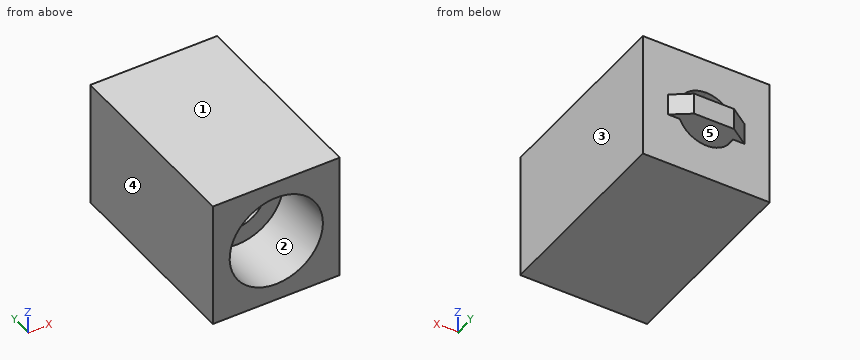
```python
from build123d import *

# Parameters (mm, degrees)
SKETCH1_R           = 12.7
BOSS_EXTRUDE1_DEPTH = 38.1
SKETCH2_R           = 5.715
CUT_EXTRUDE1_DEPTH  = 43.121134838
SKETCH3_R           = 9.3345
CUT_EXTRUDE2_DEPTH  = 12.7
SKETCH4_R           = 12.7
SKETCH4_R_2         = 5.715
BOSS_EXTRUDE2_DEPTH = 1.27
SKETCH5_W           = 11.43
SKETCH5_H           = 4.318
BOSS_EXTRUDE3_DEPTH = 6.35
BOSS_EXTRUDE4_DEPTH = 4.318
BOSS_EXTRUDE5_START = -39.37
BOSS_EXTRUDE5_DEPTH = 39.37


with BuildPart() as part:
    # Sketch1 → Boss-Extrude1 (new body)
    with BuildSketch(Plane(origin=(0, 0, 0), x_dir=(1, 0, 0), z_dir=(0, 1, 0))):
        with Locations(Location((0, 0, 0), (0, 0, 90))):
            Circle(SKETCH1_R)
    extrude(amount=BOSS_EXTRUDE1_DEPTH)

    # Sketch2 → Cut-Extrude1 (cut, through all)
    with BuildSketch(Plane(origin=(0, 38.1, 0), x_dir=(1, 0, 0), z_dir=(0, 1, 0))):
        with Locations(Location((0, 0, 0), (0, 0, 270))):
            Circle(SKETCH2_R)
    extrude(amount=-CUT_EXTRUDE1_DEPTH, mode=Mode.SUBTRACT)

    # Sketch3 → Cut-Extrude2 (cut)
    with BuildSketch(Plane.XZ):
        with Locations(Location((0, 0, 0), (0, 0, 270))):
            Circle(SKETCH3_R)
    extrude(amount=-CUT_EXTRUDE2_DEPTH, mode=Mode.SUBTRACT)

    # Sketch4 → Boss-Extrude2 (add)
    with BuildSketch(Plane(origin=(0, 38.1, 0), x_dir=(1, 0, 0), z_dir=(0, 1, 0))):
        with Locations(Location((0, 0, 0), (0, 0, 90))):
            Circle(SKETCH4_R)
        with Locations(Location((0, 0, 0), (0, 0, 270))):
            Circle(SKETCH4_R_2, mode=Mode.SUBTRACT)
    extrude(amount=BOSS_EXTRUDE2_DEPTH)

    # Sketch5 → Boss-Extrude3 (add)
    with BuildSketch(Plane(origin=(0, 39.37, 0), x_dir=(1, 0, 0), z_dir=(0, 1, 0))):
        Rectangle(SKETCH5_W, SKETCH5_H)
    extrude(amount=-BOSS_EXTRUDE3_DEPTH)

    # Sketch6 → Boss-Extrude4 (add)
    with BuildSketch(Plane(origin=(0, 0, -2.159), x_dir=(-1, 0, 0), z_dir=(0, 0, -1))):
        Polygon((7.62, 39.37), (-7.62, 39.37), (-3.992504063, 41.91), (3.992504063, 41.91), align=None)
    extrude(amount=-BOSS_EXTRUDE4_DEPTH)

    # Sketch7 → Boss-Extrude5 (add)
    with BuildSketch(Plane(origin=(0, 39.37, 0), x_dir=(1, 0, 0), z_dir=(0, 1, 0)).offset(BOSS_EXTRUDE5_START)):
        with BuildLine():
            ThreePointArc((12.7, 0), (8.980256115, -8.980256127), (-1.7e-08, -12.7))
            Line((-1.7e-08, -12.7), (12.7, -12.7))
            Line((12.7, -12.7), (12.7, 0))
        make_face()
        with BuildLine():
            ThreePointArc((-1.7e-08, -12.7), (-8.980256127, -8.980256115), (-12.7, 0))
            Line((-12.7, 0), (-12.7, -12.7))
            Line((-12.7, -12.7), (-1.7e-08, -12.7))
        make_face()
        with BuildLine():
            Line((-12.7, 12.7), (-12.7, 0))
            ThreePointArc((-12.7, 0), (-8.980256122, 8.980256121), (-1e-09, 12.7))
            Line((-1e-09, 12.7), (-12.7, 12.7))
        make_face()
        with BuildLine():
            Line((12.7, 12.7), (-1e-09, 12.7))
            ThreePointArc((-1e-09, 12.7), (8.980256121, 8.980256122), (12.7, 0))
            Line((12.7, 0), (12.7, 12.7))
        make_face()
    extrude(amount=BOSS_EXTRUDE5_DEPTH)


solid = part.part
```
Build history of the part. All positions in model axes, mm. Face numbers are marked on the shaded views. A direction names the side the tool comes from. Round coordinates to 2 decimals unless told otherwise and drop trailing zeros. Write each loop counter-clockwise with the first axis right and the second up, starting at its lowest first coordinate (ties: lowest second). Pieces come first, ordered by that corner, then holes. Notation, with made-up numbers: (67, 62) -> (95, 62) arc R15 ccw to (95, 85) -> close; hole circle Ø10 at (30.25, 43.25). An arc over 180 degrees is marked (long way). Put each result on its own line as item: value.
Item 1: Wall check: probe 1 along X at (y, z) = (28, 0) (3 decimals); probe 2 along Y at (x, z) = (2.5, 10). Give the ranges that are in metal, low to high. Write a range as from..to.
Here are the results:
probe 1: x = -12.7..-5.715, 5.715..12.7
probe 2: y = 0..39.37
Item 2: Slice it at A-A, the plane y = 35. Give the cut face in (x, z) (1 decimal), plus the area to 3 significant figures.
Here are the results:
outline: (-12.7, -12.7) -> (12.7, -12.7) -> (12.7, 12.7) -> (-12.7, 12.7) -> close; hole (-5.3, -2.2) arc R5.7 ccw to (5.3, -2.2) -> close; hole (-5.3, 2.2) -> (5.3, 2.2) arc R5.7 ccw to start
area: 591 mm^2
Item 3: Two-plate mould, pull along X, no slides. Class the marked faces 3, 4 and 5: pulls with the +X half, pulls with the -X half, needs draft (parallel to the pull), parting line crosses it, or undercut.
Here are the results:
face 3: pulls with the +X half
face 4: pulls with the -X half
face 5: undercut
Item 4: Slice it at B-B, the plane z = 0. Give the cut face in (x, y) (1 decimal), plus the area to 3 significant figures.
Here are the results:
outline: (-12.7, 0) -> (-9.3, 0) -> (-9.3, 12.7) -> (-5.7, 12.7) -> (-5.7, 33) -> (5.7, 33) -> (5.7, 12.7) -> (9.3, 12.7) -> (9.3, 0) -> (12.7, 0) -> (12.7, 39.4) -> (7.6, 39.4) -> (4, 41.9) -> (-4, 41.9) -> (-7.6, 39.4) -> (-12.7, 39.4) -> close
area: 560 mm^2
Item 5: Slice it at C-C, the plane y = 8.5. Give the cut face in (x, z), plus the area to 3 significant figures.
Here are the results:
outline: (-12.7, -12.7) -> (12.7, -12.7) -> (12.7, 12.7) -> (-12.7, 12.7) -> close; hole circle Ø18.67 at (0, 0)
area: 371 mm^2
Item 6: Tool access for the marked faces 1 and 2: list every direction of +Z, -Z, +X, -X, +Y, -Y with a clear straight run to the whole face (end or side of a thin tool).
Here are the results:
face 1: +Z, +X, -X, +Y, -Y
face 2: -Y
Item 7: Slice it at D-D, the plane x = -4.5. Give the cut face in (y, z).
Here are the results:
outline: (0, -12.7) -> (39.37, -12.7) -> (39.37, -3.52) -> (12.7, -3.52) -> (12.7, -8.18) -> (0, -8.18) -> close; (0, 8.18) -> (12.7, 8.18) -> (12.7, 3.52) -> (39.37, 3.52) -> (39.37, 12.7) -> (0, 12.7) -> close; (33.02, -2.16) -> (41.55, -2.16) -> (41.55, 2.16) -> (33.02, 2.16) -> close
Item 8: Flat gauge pins, fed straight in: P1, Ø5, axis at x = -1.5, z = 3.5, coming from the -Y side; P2, Ø10, axis at x = 10, z = -3, coming from the -Y side; P3, Ø8, axis at x = 0, z = 7, coming from the +Y side; P4, Ø3.5, axis at x = -2.5, z = -0.5, coming from the -Y side. Where does each tip first touch, or does it go through?
Here are the results:
P1: stops at y = 12.7
P2: stops at y = 0
P3: stops at y = 39.37
P4: stops at y = 33.02
